```python
from build123d import *

# Parameters (mm, degrees)
BOSS_EXTRUDE1_DEPTH = 19.05
SKETCH2_W           = 43.434
SKETCH2_H           = 13.97
MOTOR_HOLE_DEPTH    = 19.05
SKETCH3_W           = 6.35
SKETCH3_H           = 12.7
CUT_EXTRUDE2_DEPTH  = 36.941


with BuildPart() as part:
    # Sketch1 → Boss-Extrude1 (new body)
    with BuildSketch(Plane(origin=(0, 0, 0), x_dir=(1, 0, 0), z_dir=(0, 1, 0))):
        Polygon((-10.033, 66.167), (-11.6205, 66.167), (-11.6205, 76.835), (-17.9705, 76.835), (-17.9705, -78.867), (-11.6205, -78.867), (-11.6205, -66.167), (11.6205, -66.167), (11.6205, -78.867), (17.9705, -78.867), (17.9705, 76.835), (11.6205, 76.835), (11.6205, 66.167), (10.033, 66.167), (10.033, 59.817), (11.6205, 59.817), (11.6205, -59.817), (-11.6205, -59.817), (-11.6205, 59.817), (-10.033, 59.817), align=None)
    extrude(amount=BOSS_EXTRUDE1_DEPTH)

    # Sketch2 → Motor Hole (cut)
    with BuildSketch(Plane.ZY.offset(17.9705)):
        with Locations((29.972, 12.065)):
            Rectangle(SKETCH2_W, SKETCH2_H)
    extrude(amount=-MOTOR_HOLE_DEPTH, mode=Mode.SUBTRACT)

    # Sketch3 → Cut-Extrude2 (cut, through all)
    with BuildSketch(Plane.ZY.offset(17.9705)):
        with Locations((-73.66, 6.35)):
            Rectangle(SKETCH3_W, SKETCH3_H)
    extrude(amount=-CUT_EXTRUDE2_DEPTH, mode=Mode.SUBTRACT)


solid = part.part
```
Geometry check sheet. Reference: the model listing, model coordinates, mm. A direction names the side the tool comes from. Coordinates: 2 decimals unless noted, no trailing zeros. Loops run counter-clockwise (first coordinate to the right, second up) from the corner with the lowest first, then second, coordinate; pieces in that order, holes last.
Item 1: Sectioned sample at A-A, the plane y = 9. Record the boundary of the cut face in (x, z) (1 decimal), then the cut area to 3 significant figures.
Item 2: Sectioned sample at D-D, the plane z = 29.5. Record the boundary of the cut face in (x, y).
Item 3: Thickness scan on line 1 (X direction, y = 14.75, z = -60); line 2 (X direction, y = 17, z = -16.5); line 3 (Z direction, x = -11.5, y = 3.5). Record the ranges inside material, lowest first.
Item 4: Access from +Z, -Z, +X, -X, +Y, -Y to the whole of each face (thin tool, end or side, straight path). Record for faces 4 (the face through (11.62, 9, -1)), 5 (the face through (-10.033, 9, -63)), 6 (the face through (11.62, 9, 72)).
Item 5: Release check for a two-part mould opening along Z. For faces 1 (the face through (-12, 0, 3)), 2 (the face through (-15, 12, 51.689)), 3 (the face through (15, 16, -76.835)) record: released by +Z, released by -Z, zero draft, split by the parting line, or undercut.
Item 6: Go/stop test with flat-tipped pins: pin 1 Ø3 at (x, y) = (14, 4) entering from -Z (3 decimals); pin 2 Ø0.5 at (x, y) = (-11, 10) entering from +Z; pin 3 Ø5 at (x, z) = (-15, 35) entering from +Y. Record where each tip stops, or that it passes through.
Item 7: Sectioned sample at B-B, the plane z = -6. Record the boundary of the cut face in (x, y), then the cut area to 3 significant figures.
Item 8: Sectioned sample at C-C, the plane y = 2.5. Record the boundary of the cut face in (x, z) (1 decimal), then the cut area to 3 significant figures.
Check result:
1. outline: (-18, -70.5) - (-11.6, -70.5) - (-11.6, -66.2) - (-10, -66.2) - (-10, -59.8) - (-11.6, -59.8) - (-11.6, 8.3) - (-18, 8.3) - close; (-18, 51.7) - (-11.6, 51.7) - (-11.6, 59.8) - (11.6, 59.8) - (11.6, -59.8) - (10, -59.8) - (10, -66.2) - (11.6, -66.2) - (11.6, -70.5) - (18, -70.5) - (18, 78.9) - (11.6, 78.9) - (11.6, 66.2) - (-11.6, 66.2) - (-11.6, 78.9) - (-18, 78.9) - close
1. area: 1,790 mm2
2. outline: (-17.97, 0) - (-11.62, 0) - (-11.62, 5.08) - (-17.97, 5.08) - close; (11.62, 0) - (17.97, 0) - (17.97, 19.05) - (11.62, 19.05) - close
3. line 1: x = -17.97 to -10.03, 10.03 to 17.97
3. line 2: x = -17.97 to -11.62, 11.62 to 17.97
3. line 3: z = -66.17 to -59.82, 59.82 to 66.17
4. face 4: +Y, -Y
4. face 5: -Z, +Y, -Y
4. face 6: +Z, +Y, -Y
5. face 1: zero draft
5. face 2: undercut
5. face 3: released by -Z
6. pin 1: stops at z = -70.485
6. pin 2: stops at z = 66.17
6. pin 3: stops at y = 5.08
7. outline: (-17.97, 0) - (-11.62, 0) - (-11.62, 19.05) - (-17.97, 19.05) - close; (11.62, 0) - (17.97, 0) - (17.97, 19.05) - (11.62, 19.05) - close
7. area: 242 mm2
8. outline: (-18, -70.5) - (-11.6, -70.5) - (-11.6, -66.2) - (-10, -66.2) - (-10, -59.8) - (-11.6, -59.8) - (-11.6, 59.8) - (11.6, 59.8) - (11.6, -59.8) - (10, -59.8) - (10, -66.2) - (11.6, -66.2) - (11.6, -70.5) - (18, -70.5) - (18, 78.9) - (11.6, 78.9) - (11.6, 66.2) - (-11.6, 66.2) - (-11.6, 78.9) - (-18, 78.9) - close
8. area: 2,060 mm2
